For this review, take the finished solid that the model builds, in its own axes (mm). Give positions to 0.01 mm unless a question says otherwise; leave off trailing zeros.
1) For P1, Ø15, axis at x = -244, y = -194, coming from the -Z side; P2, Ø15, axis at y = -193, z = 727, coming from the +X side; P3, Ø9, axis at y = -188.5, z = 435.5, coming from the +X side, all flat-tipped, find the tip position at first contact; note any pin that passes through.
2) Draft analysis for pull direction X (two halves, no side actions). For faces 1 (the face through (665, -204.39, 320)), 2 (the face through (-917.249, 51, 451)), 3 (the face through (-210, -173.91, 624)), state which applies: pulls with the +X half, pulls with the -X half, needs draft (parallel to the pull), parting line crosses it, or undercut.
3) Wall thickness on line 1 along X through (y, z) = (-176.5, 521); line 2 along Y through (x, z) = (625.5, 634.5): over which ranges is each line inside the solid? List them lowest first.
from build123d import *

# Parameters (mm, degrees)
F0_W     = 1828.8
F0_H     = 457.2
F1_DEPTH = 914.4
F2_W     = 426.72
F2_H     = 609.6
F2_H_2   = 228.6
F3_DEPTH = 30.48


with BuildPart() as f1:
    # F0 (on Top) → F1 (new body)
    with BuildSketch(Plane.XY):
        with Locations((-2.849022, 54.689566)):
            Rectangle(F0_W, F0_H)
    extrude(amount=F1_DEPTH)

    # F2 (on face) → F3 (join)
    with BuildSketch(Plane.XZ.offset(173.910434)):
        with Locations((-673.409022, 315.940248)):
            Rectangle(F2_W, F2_H)
        with Locations((-231.449022, 315.940248)):
            Rectangle(F2_W, F2_H)
        with Locations((225.750978, 315.940248)):
            Rectangle(F2_W, F2_H)
        with Locations((667.710978, 315.940248)):
            Rectangle(F2_W, F2_H)
        with Locations((-673.409022, 765.520248)):
            Rectangle(F2_W, F2_H_2)
        with Locations((-223.829022, 765.520248)):
            Rectangle(F2_W, F2_H_2)
        with Locations((225.750978, 765.520248)):
            Rectangle(F2_W, F2_H_2)
        with Locations((675.330978, 765.520248)):
            Rectangle(F2_W, F2_H_2)
    extrude(amount=F3_DEPTH)


solid = f1.part
Results list:
1. P1: stops at z = 11.14
1. P2: stops at x = 888.69
1. P3: stops at x = 881.07
2. face 1: needs draft
2. face 2: pulls with the -X half
2. face 3: undercut
3. line 1: x = -886.77 to -460.05, -444.81 to -18.09, 12.39 to 439.11, 454.35 to 881.07
3. line 2: y = -173.91 to 283.29
